```python
from build123d import *

# Parameters (mm, degrees)
SKETCH1_W           = 76.2
SKETCH1_H           = 3.175
BOSS_EXTRUDE1_DEPTH = 69.85
SKETCH2_W           = 12.7
SKETCH2_H           = 6.35
CUT_EXTRUDE1_DEPTH  = 439.214737942


with BuildPart() as part:
    # Sketch1 → Boss-Extrude1 (new body)
    with BuildSketch(Plane.XY):
        with Locations((-394.500339141, 196.359630659)):
            Rectangle(SKETCH1_W, SKETCH1_H)
    extrude(amount=-BOSS_EXTRUDE1_DEPTH)

    # Sketch2 → Cut-Extrude1 (cut, through all)
    with BuildSketch(Plane(origin=(0, 197.947130659, 0), x_dir=(1, 0, 0), z_dir=(0, 1, 0))):
        with Locations((-362.750339141, 3.175)):
            Rectangle(SKETCH2_W, SKETCH2_H)
        with Locations((-394.500339141, 3.175)):
            Rectangle(SKETCH2_W, SKETCH2_H)
        with Locations((-426.250339141, 3.175)):
            Rectangle(SKETCH2_W, SKETCH2_H)
        with Locations((-362.750339141, 66.675)):
            Rectangle(SKETCH2_W, SKETCH2_H)
        with Locations((-394.500339141, 66.675)):
            Rectangle(SKETCH2_W, SKETCH2_H)
        with Locations((-426.250339141, 66.675)):
            Rectangle(SKETCH2_W, SKETCH2_H)
    extrude(amount=-CUT_EXTRUDE1_DEPTH, mode=Mode.SUBTRACT)


solid = part.part
```
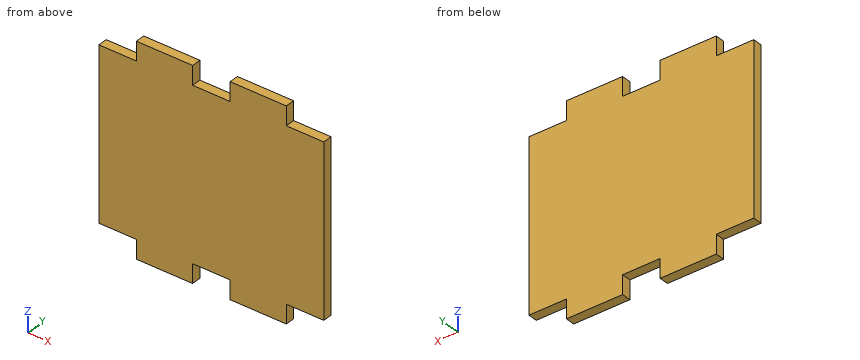
Check sheet for the modelled part. Datum: model origin and axes. Units: mm. Give positions to 0.01 mm unless a question says otherwise; leave off trailing zeros. Order: outer loops, then holes, each group sorted by start corner. A loop starts at its lowest first (then second) coordinate and runs counter-clockwise, first axis right, second up. Notation, with made-up numbers: M 35,49.5 L 83,49.5 A6 cw 83,59.5 Z; hole C -29.75,14.5 d3. An arc over 180 degrees is marked long. Answer in a Markdown table with one row per item. Add a question column.
Q1. Sectioned sample at B-B, the plane y = 195.25. Record the boundary of the cut face in (x, z), and give its area (3 significant figures).
Q2. Sectioned sample at C-C, the plane x = -421. Record the boundary of the cut face in (y, z), and give its area (3 significant figures).
Q3. Gauge pin test, flat ends, axial feed: pin 1 Ø1.6 at (x, y) = (-397, 196) entering from +Z; pin 2 Ø1 at (x, y) = (-424, 196) entering from -Z; pin 3 Ø1 at (y, z) = (197, -65.5) entering from -X. Record the tip position at first contact, or that the pin passes through.
Q4. Sectioned sample at A-A, the plane z = -3.5. Record the boundary of the cut face in (x, y), and give its area (3 significant figures).
Q5. Thickness scan on L1, parallel to Z at x = -361, y = 196.25. Record the ranges inside material, lowest first.
Verdict:
| question | item | result |
|---|---|---|
| 1 | outline | M -432.6,-63.5 L -419.9,-63.5 L -419.9,-69.85 L -400.85,-69.85 L -400.85,-63.5 L -388.15,-63.5 L -388.15,-69.85 L -369.1,-69.85 L -369.1,-63.5 L -356.4,-63.5 L -356.4,-6.35 L -369.1,-6.35 L -369.1,0 L -388.15,0 L -388.15,-6.35 L -400.85,-6.35 L -400.85,0 L -419.9,0 L -419.9,-6.35 L -432.6,-6.35 Z |
| 1 | area | 4,840 mm² |
| 2 | outline | M 194.77,-63.5 L 197.95,-63.5 L 197.95,-6.35 L 194.77,-6.35 Z |
| 2 | area | 181 mm² |
| 3 | pin 1 | z = -6.35 |
| 3 | pin 2 | z = -63.5 |
| 3 | pin 3 | x = -419.9 |
| 4 | outline | M -419.9,194.77 L -400.85,194.77 L -400.85,197.95 L -419.9,197.95 Z; M -388.15,194.77 L -369.1,194.77 L -369.1,197.95 L -388.15,197.95 Z |
| 4 | area | 121 mm² |
| 5 | L1 | -63.5 to -6.35 |
